```python
from build123d import *

# Parameters (mm, degrees)
F0_W     = 28.194
F0_H     = 28.194
F1_DEPTH = 28.194
F2_R     = 6.477
F3_DEPTH = 28.195
F4_R     = 53.155015
F5_DEPTH = 25.4
F6_R     = 52.277652
F7_DEPTH = 25.4


with BuildPart() as f1:
    # F0 (on Front) → F1 (new body)
    with BuildSketch(Plane.XZ):
        with Locations((-14.097, -14.097)):
            Rectangle(F0_W, F0_H)
    extrude(amount=F1_DEPTH)

    # F2 (on face) → F3 (cut, through all)
    with BuildSketch(Plane.YZ):
        with Locations((-12.954, -12.954)):
            Circle(F2_R)
    extrude(amount=-F3_DEPTH, mode=Mode.SUBTRACT)

    # F4 (on face) → F5 (join)
    with BuildSketch(Plane.YZ):
        with Locations((-12.954, -12.954)):
            Circle(F4_R)
    extrude(amount=F5_DEPTH)

    # F6 (on face) → F7 (join)
    with BuildSketch(Plane(origin=(-28.194, 0, 0), x_dir=(0, -1, 0), z_dir=(-1, 0, 0))):
        with Locations((12.954, -12.954)):
            Circle(F6_R)
    extrude(amount=F7_DEPTH)


solid = f1.part
```
Check sheet for the modelled part. Datum: model origin and axes. Units: mm. A direction names the side the tool comes from. Give positions to 0.01 mm unless a question says otherwise; leave off trailing zeros. Write each loop counter-clockwise with the first axis right and the second up, starting at its lowest first coordinate (ties: lowest second). Pieces come first, ordered by that corner, then holes.
Item 1: Access from +Z, -Z, +X, -X, +Y, -Y to the whole of each face (thin tool, end or side, straight path). Record for faces 4 (the face through (-14, -14, -28.194)), 5 (the face through (-14, -28.194, -14)), 6 (the face through (-14, -14, 0)), 7 (the face through (0, -14, -36)).
Item 2: Cross-section at C-C (z = -11.5). Enter the section's corners in (x, y), and give its area (3 significant figures).
Item 3: Scan lines: L1, parallel to X at y = -44.5, z = 7; L2, parallel to Y at x = -9, z = -7.5; L3, parallel to Z at x = -8.5, y = -10. Record each from-to range of solid material in increasing order.
Item 4: Cross-section at D-D (x = -30.5). Enter the section's corners in (y, z).
Item 5: Draft check along X on faces 1 (the face through (12.522, -55.136, -45.298)), 2 (the face through (-28.194, -13, -13)), 3 (the face through (-53.594, -12, -12)). Enter one of: released by +X, released by -X, zero draft, split by the parting line, or undercut.
Item 6: Gauge pin test, flat ends, axial feed: pin 1 (22.5 mm diameter, centred on x = -15, z = -16.5, fed in from +Y); pin 2 (14 mm diameter, centred on x = -18, y = -15, fed in from +Z); pin 3 (10 mm diameter, centred on x = -35, z = -18, fed in from -Y). Record the tip position at first contact, or that the pin passes through.
Item 7: Cross-section at A-A (z = -51.5). Enter the section's corners in (x, y).
Item 8: Cross-section at B-B (y = 7). Enter the section's corners in (x, z).
Report:
1. face 4: -Z, +Y, -Y
1. face 5: +Z, -Z, -Y
1. face 6: +Z, +Y, -Y
1. face 7: none
2. outline: (-53.59, -65.21) - (-28.19, -65.21) - (-28.19, -28.19) - (0, -28.19) - (0, -66.09) - (25.4, -66.09) - (25.4, 40.18) - (0, 40.18) - (0, 0) - (-28.19, 0) - (-28.19, 39.3) - (-53.59, 39.3) - close; hole (-28.19, -19.27) - (0, -19.27) - (0, -6.64) - (-28.19, -6.64) - close
2. area: 5,790 mm2
3. L1: x = -53.59 to -28.19, 0 to 25.4
3. L2: y = -28.19 to -16.45, -9.46 to 0
3. L3: z = -28.19 to -18.72, -7.19 to 0
4. outline: circle Ø104.56 at (-12.95, -12.95)
5. face 1: zero draft
5. face 2: undercut
5. face 3: released by -X
6. pin 1: stops at y = 0
6. pin 2: stops at z = 0
6. pin 3: stops at y = -65.23
7. outline: (-53.59, -48.27) - (-28.19, -48.27) - (-28.19, 22.36) - (-53.59, 22.36) - close; (0, -49.56) - (25.4, -49.56) - (25.4, 23.65) - (0, 23.65) - close
8. outline: (-53.59, -61.27) - (-28.19, -61.27) - (-28.19, 35.37) - (-53.59, 35.37) - close; (0, -62.22) - (25.4, -62.22) - (25.4, 36.31) - (0, 36.31) - close
